Check sheet for the modelled part. Datum: model origin and axes. Units: mm. A direction names the side the tool comes from. Round coordinates to 2 decimals unless told otherwise and drop trailing zeros. Loops run counter-clockwise (first coordinate to the right, second up) from the corner with the lowest first, then second, coordinate; pieces in that order, holes last. Notation, with made-up numbers: (-13, 8.25) -> (35, 8.25) arc R14 ccw to (35, 13.25) -> close; hole circle Ø7 at (27.5, 66). An arc over 180 degrees is marked (long way). Use one line per item in the form item = value. Start each with the question number.
(1) Sectioned sample at B-B (z = 10.5). Record the cut outline in (x, y), and give its area (3 significant figures).
(2) Sectioned sample at A-A (y = -1.5). Record the cut outline in (x, z), and give its area (3 significant figures).
(3) Sectioned sample at C-C (x = -16). Record the cut outline in (y, z), and give its area (3 significant figures).
(4) Set-up check for faces 4 (the flat face through (-37.235, -1, -1)), 5 (the flat face through (-17.235, 1, 11)), 6 (the flat face through (2, 13.258, 8)), 7 (the flat face through (-5, -11.742, 11)), 8 (the flat face through (-5, -4, 7)): record each of +Z, -Z, +X, -X, +Y, -Y from which the full face is reachable in a straight line by a thin tool's end or side.
(5) Material ranges on probe 1 along X at (y, z) = (-1.75, 11); probe 2 along Z at (x, y) = (-26, 3); probe 3 along Y at (x, z) = (-15, 18.5), recorded low to high. Write a range as [from, to].
(6) Sectioned sample at D-D (y = -13). Record the cut outline in (x, z).
(7) Draft check along Y on faces 1 (the flat face through (7.765, 1, 11)), 2 (the flat face through (13, -14.742, -1)), 3 (the flat face through (-5, 6, 7)). Enter one of: released by +Y, released by -Y, zero draft, split by the parting line, or undercut.
(8) Go/stop test with flat-tipped pins: pin 1 (1 mm diameter, centred on y = 0.5, z = 16, fed in from +X); pin 2 (5 mm diameter, centred on x = 21.5, y = -9, fed in from +Z); pin 3 (11 mm diameter, centred on y = 5.5, z = 15.5, fed in from -X). Record where each tip stops, or that it passes through.
from build123d import *

# Parameters (mm, degrees)
ESQUISSE1_W             = 25
ESQUISSE1_H             = 25
BOSS_EXTRU_1_DEPTH      = 22
ESQUISSE2_R             = 1.25
ENL_V_MAT_EXTRU_1_DEPTH = 15
ESQUISSE3_W             = 100
ESQUISSE3_H             = 28
BOSS_EXTRU_2_DEPTH      = 3


with BuildPart() as part:
    # Esquisse1 → Boss.-Extru.1 (new body)
    with BuildSketch(Plane.XY):
        with Locations((-4.734848485, 0.757575758)):
            Rectangle(ESQUISSE1_W, ESQUISSE1_H)
    extrude(amount=BOSS_EXTRU_1_DEPTH)

    # Esquisse2 → Enlèv. mat.-Extru.1 (cut)
    with BuildSketch(Plane.XY.offset(22)):
        with Locations((-4.734848485, 5.757575758)):
            Circle(ESQUISSE2_R)
        with Locations((-4.734848485, -4.242424242)):
            Circle(ESQUISSE2_R)
    extrude(amount=-ENL_V_MAT_EXTRU_1_DEPTH, mode=Mode.SUBTRACT)

    # Esquisse3 → Boss.-Extru.2 (add)
    with BuildSketch(Plane(origin=(0, 0, 0), x_dir=(-1, 0, 0), z_dir=(0, 0, -1))):
        with Locations((-12.765151515, -0.742424242)):
            Rectangle(ESQUISSE3_W, ESQUISSE3_H)
    extrude(amount=BOSS_EXTRU_2_DEPTH)


solid = part.part
Checks:
q1.outline = (-17.23, -11.74) -> (7.77, -11.74) -> (7.77, 13.26) -> (-17.23, 13.26) -> close; hole circle Ø2.5 at (-4.73, -4.24); hole circle Ø2.5 at (-4.73, 5.76)
q1.area = 615 mm2
q2.outline = (-37.23, -3) -> (62.77, -3) -> (62.77, 0) -> (7.77, 0) -> (7.77, 22) -> (-17.23, 22) -> (-17.23, 0) -> (-37.23, 0) -> close
q2.area = 850 mm2
q3.outline = (-14.74, -3) -> (13.26, -3) -> (13.26, 22) -> (-11.74, 22) -> (-11.74, 0) -> (-14.74, 0) -> close
q3.area = 634 mm2
q4.face_4 = +Z, -Z, -X, +Y, -Y
q4.face_5 = +Z, -X, +Y, -Y
q4.face_6 = +Z, -Z, +X, -X, +Y
q4.face_7 = +Z, +X, -X, -Y
q4.face_8 = +Z
q5.probe_1 = [-17.23, 7.77]
q5.probe_2 = [-3, 0]
q5.probe_3 = [-11.74, 13.26]
q6.outline = (-37.23, -3) -> (62.77, -3) -> (62.77, 0) -> (-37.23, 0) -> close
q7.face_1 = zero draft
q7.face_2 = released by -Y
q7.face_3 = undercut
q8.pin_1 = 7.77
q8.pin_2 = 0
q8.pin_3 = -17.23
